```python
from build123d import *

# Parameters (mm, degrees)
EXTRUDE_2_DEPTH     = 2
EXTRUDE_4_DEPTH     = 1
SKETCH_7_W          = 0.8
SKETCH_7_H          = 10
EXTRUDE_8_DEPTH     = 2.8
SKETCH_8_R          = 0.75
EXTRUDE_9_DEPTH     = 10
FILLET_1_R          = 0.85
SKETCH_11_W         = 1
SKETCH_11_H         = 1
CUT_EXTRUDE_1_DEPTH = 1.2
FILLET_2_R          = 1
SKETCH_13_W         = 0.8
SKETCH_13_H         = 10
EXTRUDE_10_DEPTH    = 1.8
SKETCH_14_R         = 0.75
EXTRUDE_11_DEPTH    = 10
FILLET_3_R          = 0.85
SKETCH_15_W         = 0.8
SKETCH_15_H         = 1
CUT_EXTRUDE_3_DEPTH = 1
FILLET_4_R          = 1


# Some blends are built 0.0001 mm under size
with BuildPart() as part:
    # case 2 → 凸台-拉伸2 (new body)
    with BuildSketch(Plane(origin=(0, 0, 0), x_dir=(1, 0, 0), z_dir=(0, 1, 0))):
        with BuildLine():
            Line((-51.542196447, 13), (-51.542196447, 18))
            Line((-51.542196447, 18), (-46.542196447, 18))
            Line((-46.542196447, 18), (43.457803553, 18))
            Line((43.457803553, 18), (48.457803553, 18))
            Line((48.457803553, 18), (48.457803553, 13))
            Line((48.457803553, 13), (48.457803553, -13))
            ThreePointArc((48.457803553, -13), (46.993337459, -16.535533906), (43.457803553, -18))
            Line((43.457803553, -18), (-46.542196447, -18))
            ThreePointArc((-46.542196447, -18), (-50.077730353, -16.535533906), (-51.542196447, -13))
            Line((-51.542196447, -13), (-51.542196447, 13))
        make_face()
    extrude(amount=EXTRUDE_2_DEPTH)

    # 草图3 → 凸台-拉伸4 (add)
    with BuildSketch(Plane(origin=(0, 2, 0), x_dir=(1, 0, 0), z_dir=(0, 1, 0))):
        with BuildLine():
            Line((-49.392196447, 13), (-49.392196447, -13))
            ThreePointArc((-49.392196447, -13), (-48.452846076, -14.910649629), (-46.542196447, -15.85))
            Line((-46.542196447, -15.85), (43.457803553, -15.85))
            ThreePointArc((43.457803553, -15.85), (45.368453181, -14.910649629), (46.307803553, -13))
            Line((46.307803553, -13), (46.307803553, 13))
            ThreePointArc((46.307803553, 13), (45.368453181, 14.910649629), (43.457803553, 15.85))
            Line((43.457803553, 15.85), (-46.542196447, 15.85))
            ThreePointArc((-46.542196447, 15.85), (-48.452846076, 14.910649629), (-49.392196447, 13))
        make_face()
        with BuildLine():
            Line((-46.542196447, -15.05), (43.457803553, -15.05))
            ThreePointArc((43.457803553, -15.05), (44.827315928, -14.369512375), (45.507803553, -13))
            Line((45.507803553, -13), (45.507803553, 13))
            ThreePointArc((45.507803553, 13), (44.827315928, 14.369512375), (43.457803553, 15.05))
            Line((43.457803553, 15.05), (-46.542196447, 15.05))
            ThreePointArc((-46.542196447, 15.05), (-47.911708823, 14.369512375), (-48.592196447, 13))
            Line((-48.592196447, 13), (-48.592196447, -13))
            ThreePointArc((-48.592196447, -13), (-47.911708823, -14.369512375), (-46.542196447, -15.05))
        make_face(mode=Mode.SUBTRACT)
    extrude(amount=EXTRUDE_4_DEPTH)

    # 草图7 → 凸台-拉伸8 (add)
    with BuildSketch(Plane(origin=(0, 2, 0), x_dir=(1, 0, 0), z_dir=(0, 1, 0))):
        with Locations((-48.992196447, 0)):
            Rectangle(SKETCH_7_W, SKETCH_7_H)
    extrude(amount=EXTRUDE_8_DEPTH)

    # 草图8 → 凸台-拉伸9 (add)
    with BuildSketch(Plane.XY.offset(5)):
        with Locations((-49.392196447, 3.6)):
            Circle(SKETCH_8_R)
    extrude(amount=-EXTRUDE_9_DEPTH)

    # 圆角1
    # the kernel refuses this fillet: 0.85 mm, written as the material it takes off along each edge
    with BuildSketch(Plane(origin=(-49.392196447, 4.8, 6.875), x_dir=(0, -1, 0), z_dir=(0, 0, -1))) as fillet_1_piece_1:
        with BuildLine():
            CenterArc((0.85, -0.75), FILLET_1_R, 118.072486936, 61.927513064)
            Line((0, -0.75), (-0.017, -0.75))
            Line((-0.017, -0.75), (-0.017, 0))
            Line((-0.017, 0), (0, 0.017))
            ThreePointArc((0, 0.017), (0.225, 0.017), (0.442, 0.015))
            Line((0.442, 0.015), (0.45, 0))
        make_face()
    extrude(amount=13.75, mode=Mode.SUBTRACT)

    # 草图11 → 切除-拉伸1 (cut)
    with BuildSketch(Plane.ZY.offset(49.392196447)):
        with Locations((5.5, 2.5)):
            Rectangle(SKETCH_11_W, SKETCH_11_H)
        with Locations((-5.5, 2.5)):
            Rectangle(SKETCH_11_W, SKETCH_11_H)
    extrude(amount=-CUT_EXTRUDE_1_DEPTH, mode=Mode.SUBTRACT)

    # 圆角2
    fillet_2_edges = [part.edges().sort_by_distance(p)[0] for p in [
        (-48.992196447, 3, 6),
        (-48.992196447, 3, -6),
    ]]
    fillet(fillet_2_edges, radius=FILLET_2_R - 0.0001)  # a hair under: the kernel refuses the full size

    # 草图13 → 凸台-拉伸10 (add)
    with BuildSketch(Plane(origin=(0, 3, 0), x_dir=(1, 0, 0), z_dir=(0, 1, 0))):
        with Locations((45.907803553, 0)):
            Rectangle(SKETCH_13_W, SKETCH_13_H)
    extrude(amount=EXTRUDE_10_DEPTH)

    # 草图14 → 凸台-拉伸11 (add)
    with BuildSketch(Plane.XY.offset(5)):
        with Locations((46.307803553, 3.6)):
            Circle(SKETCH_14_R)
    extrude(amount=-EXTRUDE_11_DEPTH)

    # 圆角3
    # the kernel refuses this fillet: 0.85 mm, written as the material it takes off along each edge
    with BuildSketch(Plane(origin=(46.307803553, 4.8, -6.875), x_dir=(0, -1, 0), z_dir=(0, 0, 1))) as fillet_3_piece_1:
        with BuildLine():
            CenterArc((0.85, -0.75), FILLET_3_R, 118.072486936, 61.927513064)
            Line((0, -0.75), (-0.017, -0.75))
            Line((-0.017, -0.75), (-0.017, 0))
            Line((-0.017, 0), (0, 0.017))
            ThreePointArc((0, 0.017), (0.225, 0.017), (0.442, 0.015))
            Line((0.442, 0.015), (0.45, 0))
        make_face()
    extrude(amount=13.75, mode=Mode.SUBTRACT)

    # 草图15 → 切除-拉伸3 (cut)
    with BuildSketch(Plane(origin=(0, 3, 0), x_dir=(1, 0, 0), z_dir=(0, 1, 0))):
        with Locations((45.907803553, 5.5)):
            Rectangle(SKETCH_15_W, SKETCH_15_H)
        with Locations((45.907803553, -5.5)):
            Rectangle(SKETCH_15_W, SKETCH_15_H)
    extrude(amount=-CUT_EXTRUDE_3_DEPTH, mode=Mode.SUBTRACT)

    # 圆角4
    fillet_4_edges = [part.edges().sort_by_distance(p)[0] for p in [
        (45.907803553, 3, 6),
        (45.907803553, 3, -6),
    ]]
    fillet(fillet_4_edges, radius=FILLET_4_R - 0.0001)  # a hair under: the kernel refuses the full size


solid = part.part
```
Input: part model. Units: mm. Frame: model coordinates. A direction names the side the tool comes from. Give positions to 0.01 mm unless a question says otherwise; leave off trailing zeros. Order: outer loops, then holes, each group sorted by start corner. A loop starts at its lowest first (then second) coordinate and runs counter-clockwise, first axis right, second up. Notation, with made-up numbers: (26.5, 60) - (43.5, 60) arc R13 ccw to (43.5, 66) - close; hole circle Ø1 at (2, 87.25). An arc over 180 degrees is marked (long way). One line per item, written item: value.
1. Pin query (flat end, axial travel): pin 1 Ø11 at (x, z) = (13, -3.5) entering from +Y; pin 2 Ø0.8 at (y, z) = (2.5, -10) entering from -X; pin 3 Ø1.2 at (x, y) = (46.5, 3) entering from -Z. Return the tip coordinate at first contact, or that it passes through.
Determined:
pin 1: y = 2
pin 2: x = -49.39
pin 3: z = -14.21
2. Cut plane A-A, the plane z = 8. Output: boundary loops of the cut face in (x, y), and give its area (3 significant figures).
Determined:
outline: (-51.54, 0) - (48.46, 0) - (48.46, 2) - (46.31, 2) - (46.31, 3) - (45.51, 3) - (45.51, 2) - (-48.59, 2) - (-48.59, 3) - (-49.39, 3) - (-49.39, 2) - (-51.54, 2) - close
area: 202 mm2
3. Draft query along X for faces 6 (the face through (-50.039, 0.986, 16.574)), 7 (the face through (-1, 0, 0)), 8 (the face through (45.35, 2.49, 14.93)), 9 (the face through (-47.9, 2.49, -14.38)). Return one class per face: released by +X, released by -X, zero draft, split by the parting line, or undercut.
Determined:
face 6: released by -X
face 7: zero draft
face 8: released by +X
face 9: undercut
4. Line query: probe 1 along X at (y, z) = (2.4, 11.5); probe 2 along Z at (x, y) = (-17.5, 2.1); probe 3 along X at (y, z) = (3.5, -3). Output: solid intervals per line, ascending.
Determined:
probe 1: -49.39 to -48.59, 45.51 to 46.31
probe 2: -15.85 to -15.05, 15.05 to 15.85
probe 3: -50.14 to -48.59, 45.51 to 47.05
5. Reachability of faces 1 (the face through (44.843, 2.493, -14.354)), 2 (the face through (-48.474, 2.493, 14.889)), 3 (the face through (-2, 1, -18)), 4 (the face through (-48.431, 2.493, -14.932)), 5 (the face through (45.39, 2.49, -14.89)) from +Z, -Z, +X, -X, +Y, -Y: full face, straight path, thin tool, end or side. Return the list, or none.
Determined:
face 1: +Y
face 2: +Z, -X, +Y
face 3: -Z, +X, -X, +Y, -Y
face 4: -Z, -X, +Y
face 5: -Z, +X, +Y
6. Cut plane B-B, the plane x = 5. Output: boundary loops of the cut face in (y, z), and give its area (3 significant figures).
Determined:
outline: (0, -18) - (2, -18) - (2, -15.85) - (3, -15.85) - (3, -15.05) - (2, -15.05) - (2, 15.05) - (3, 15.05) - (3, 15.85) - (2, 15.85) - (2, 18) - (0, 18) - close
area: 73.6 mm2
